Source: CAD feature listing. Evaluate the final solid. Frame: model axes, mm. Face numbers are marked on the shaded views. A direction names the side the tool comes from. Round coordinates to 2 decimals unless told otherwise and drop trailing zeros. Loops run counter-clockwise (first coordinate to the right, second up) from the corner with the lowest first, then second, coordinate; pieces in that order, holes last.
(1) Section A-A, the plane z = 7. Return the cut outline in (x, y), plus the area to 3 significant figures.
(2) Section B-B, the plane x = 5.5. Return the cut outline in (y, z), plus the area to 3 significant figures.
(3) First-contact query: pin 1 Ø1.5 at (x, y) = (4, -17) entering from -Z; pin 2 Ø1.5 at (x, z) = (4.5, 11) entering from -Y. Flat tips, straight axial feed; report the tip coordinate or a pass-through.
(4) Section D-D, the plane y = -3.5. Return the cut outline in (x, z), plus the area to 3 significant figures.
(5) Set-up query: the marked faces 1, 2 and 3. Return all of +Z, -Z, +X, -X, +Y, -Y with unobstructed straight access to the full face (end or side cutting, diameter ignored); none if empty.
(6) Section C-C, the plane z = 3. Return the cut outline in (x, y).
(7) Material intervals for probe 1 along Y at (x, z) = (5.35, 11); probe 2 along Z at (x, y) = (3.9, -11); probe 3 along Z at (x, y) = (4.65, -3.25), sorted ascending.
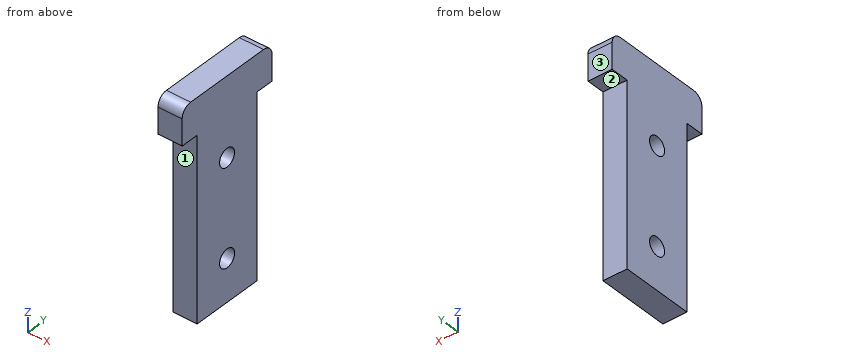
```python
from build123d import *

# Parameters (mm, degrees)
F0_R     = 1.5
F1_DEPTH = 4
F2_ANGLE = 90
F4_ANGLE = 90


with BuildPart() as f1:
    # F0 (on Top) → F1 (new body)
    with BuildSketch(Plane.XY):
        with BuildLine():
            Line((-6, 13.9288183318), (-6, -16.0711816682))
            Line((-6, -16.0711816682), (6, -16.0711816682))
            Line((6, -16.0711816682), (6, 13.9288183318))
            Line((6, 13.9288183318), (9, 13.9288183318))
            Line((9, 13.9288183318), (9, 18.2345626692))
            ThreePointArc((9, 18.2345626692), (8.5037640055, 19.4325823373), (7.3057443374, 19.9288183318))
            Line((7.3057443374, 19.9288183318), (-7.3057443374, 19.9288183318))
            ThreePointArc((-7.3057443374, 19.9288183318), (-8.5037640055, 19.4325823373), (-9, 18.2345626692))
            Line((-9, 18.2345626692), (-9, 13.9288183318))
            Line((-9, 13.9288183318), (-6, 13.9288183318))
        make_face()
        with Locations((0, -9.0711816682)):
            Circle(F0_R, mode=Mode.SUBTRACT)
        with Locations((0, 6.9308183318)):
            Circle(F0_R, mode=Mode.SUBTRACT)
    extrude(amount=F1_DEPTH)


with BuildPart() as f1_1:
    # F2: moved
    add(f1.part.rotate(Axis((0, -16.0711816682, 0), (1, 0, 0)), F2_ANGLE))


with BuildPart() as f1_2:
    # F4: moved
    add(f1_1.part.rotate(Axis((6, -16.0711816682, 1.3093175367), (0, 0, -1)), F4_ANGLE))


solid = f1_2.part
```
Output values:
1. outline: (2, -16.07) - (6, -16.07) - (6, -11.57) - (2, -11.57) - close; (2, -8.57) - (6, -8.57) - (6, -4.07) - (2, -4.07) - close
1. area: 36.0 mm2
2. outline: (-19.07, 30) - (-16.07, 30) - (-16.07, 0) - (-4.07, 0) - (-4.07, 30) - (-1.07, 30) - (-1.07, 34.31) arc R1.69 ccw to (-2.77, 36) - (-17.38, 36) arc R1.69 ccw to (-19.07, 34.31) - close; hole circle Ø3 at (-10.07, 7); hole circle Ø3 at (-10.07, 23)
2. area: 453 mm2
3. pin 1: stops at z = 30
3. pin 2: stops at y = -16.07
4. outline: (2, 30) - (6, 30) - (6, 36) - (2, 36) - close
4. area: 24.0 mm2
5. face 1: -Z, +X, -X, -Y
5. face 2: -Z, +X, -X, +Y
5. face 3: +Z, -Z, +X, -X, +Y
6. outline: (2, -16.07) - (6, -16.07) - (6, -4.07) - (2, -4.07) - close
7. probe 1: y = -16.07 to -4.07
7. probe 2: z = 0 to 5.82, 8.18 to 21.82, 24.18 to 36
7. probe 3: z = 30 to 36
